from build123d import *

# Parameters (mm, degrees)
F0_R      = 6
F1_DEPTH  = 1
F2_R      = 12
F2_R_2    = 6
F3_DEPTH  = 10.5
F5_DEPTH  = 10.5
F6_R      = 4
F7_DEPTH  = 6.5
F8_R      = 3
F9_DEPTH  = 8.382
F10_W     = 2.7
F10_H     = 0.5
F11_DEPTH = 3.5
F12_R     = 16.3576
F13_DEPTH = 16.51


with BuildPart() as f1:
    # F0 (on Top) → F1 (new body)
    with BuildSketch(Plane.XY):
        Circle(F0_R)
    extrude(amount=-F1_DEPTH)

    # F2 (on face) → F3 (join)
    with BuildSketch(Plane(origin=(0, 0, -1), x_dir=(1, 0, 0), z_dir=(0, 0, -1))):
        Circle(F2_R)
        Circle(F2_R_2, mode=Mode.SUBTRACT)
        Circle(F2_R_2)
    extrude(amount=F3_DEPTH)

    # F4 (on face) → F5 (join, through all)
    with BuildSketch(Plane.XY.offset(-1)):
        with BuildLine():
            Line((6.35, 9), (6.35, -9))
            Line((6.35, -9), (7.9372539332, -9))
            ThreePointArc((7.9372539332, -9), (10.9372539332, -4.9372539332), (12, 0))
            ThreePointArc((12, 0), (10.9372539332, 4.9372539332), (7.9372539332, 9))
            Line((7.9372539332, 9), (6.35, 9))
        make_face()
        with BuildLine():
            ThreePointArc((12, 0), (10.9372539332, -4.9372539332), (7.9372539332, -9))
            Line((7.9372539332, -9), (20, -9))
            Line((20, -9), (20, 9))
            Line((20, 9), (7.9372539332, 9))
            ThreePointArc((7.9372539332, 9), (10.9372539332, 4.9372539332), (12, 0))
        make_face()
    extrude(amount=-F5_DEPTH)

    # F6 (on face) → F7 (join)
    with BuildSketch(Plane.XY):
        Circle(F6_R)
    extrude(amount=F7_DEPTH)

    # F8 (on face) → F9 (join)
    with BuildSketch(Plane.XY.offset(6.5)):
        Circle(F8_R)
    extrude(amount=F9_DEPTH)

    # F10 (on face) → F11 (join)
    with BuildSketch(Plane.XY.offset(-1)):
        with Locations((0, -12)):
            Rectangle(F10_W, F10_H)
    extrude(amount=F11_DEPTH)

    # F12 (on face) → F13 (join)
    with BuildSketch(Plane.XY.offset(6.5)):
        Circle(F12_R)
    extrude(amount=F13_DEPTH)


solid = f1.part
Check sheet for the modelled part. Datum: model origin and axes. Units: mm. A direction names the side the tool comes from. Round coordinates to 2 decimals unless told otherwise and drop trailing zeros. Loops run counter-clockwise (first coordinate to the right, second up) from the corner with the lowest first, then second, coordinate; pieces in that order, holes last. Notation, with made-up numbers: (59, -33) - (81, -33) arc R13 ccw to (81, -23) - close; hole circle Ø10 at (29.25, -7). An arc over 180 degrees is marked (long way). Answer as CSV lines item,"result". Start each with the question number.
Item 1: Section check B-B (y = -11). Record the boundary of the cut face in (x, z), and give its area (3 significant figures).
Item 2: Section check C-C (x = 0.5). Record the boundary of the cut face in (y, z).
Item 3: Section check D-D (x = 6.5). Record the boundary of the cut face in (y, z), and give its area (3 significant figures).
Item 4: Section check A-A (y = 0). Record the boundary of the cut face in (x, z).
Item 5: Release check for a two-part mould opening along Z. For faces 5 (the flat face through (-1.42, -3.92, 0)), 6 (the flat face through (0, 0, 23.01)), 7 (the flat face through (4, 0, -11.5)) record: +Z half, -Z half, draft (parallel to the pull), parting line (faces both ways), or undercut.
Item 6: Scan lines: line 1 (Z direction, x = -5, y = 1.5); line 2 (Z direction, x = 13.5, y = 6.5); line 3 (Z direction, x = 0, y = 13). Record each from-to range of solid material in increasing order. Write a range as [from, to].
Item 7: Set-up check for faces 1 (the flat face through (0, -12.25, 1)), 2 (the cylindrical face through (-12, 0, -6)), 3 (the cylindrical face through (15.602, 4.913, 14.639)), 4 (the cylindrical face through (-5.994, 0.264, -0.493)): record each of +Z, -Z, +X, -X, +Y, -Y from which the full face is reachable in a straight line by a thin tool's end or side.
Item 8: Depth check by flat-ended pin: P1, Ø2, axis at x = 0, z = 1.5, coming from the +Y side; P2, Ø3, axis at x = 13.5, z = -6, coming from the -Y side; P3, Ø8.5, axis at x = 12, z = -6.5, coming from the +Y side. Enter the tip coordinate at first touch or a pass-through.
Report:
1,outline,"(-12.11, 6.5) - (12.11, 6.5) - (12.11, 23.01) - (-12.11, 23.01) - close; (-4.8, -11.5) - (4.8, -11.5) - (4.8, -1) - (-4.8, -1) - close"
1,area,"500 mm2"
2,outline,"(-16.35, 6.5) - (-3.97, 6.5) - (-3.97, 0) - (-5.98, 0) - (-5.98, -1) - (-11.75, -1) - (-11.75, 2.5) - (-12.25, 2.5) - (-12.25, -1) - (-11.99, -1) - (-11.99, -11.5) - (11.99, -11.5) - (11.99, -1) - (5.98, -1) - (5.98, 0) - (3.97, 0) - (3.97, 6.5) - (16.35, 6.5) - (16.35, 23.01) - (-16.35, 23.01) - close"
3,outline,"(-15.01, 6.5) - (15.01, 6.5) - (15.01, 23.01) - (-15.01, 23.01) - close; (-10.09, -11.5) - (10.09, -11.5) - (10.09, -1) - (-10.09, -1) - close"
3,area,"707 mm2"
4,outline,"(-16.36, 6.5) - (-4, 6.5) - (-4, 0) - (-6, 0) - (-6, -1) - (-12, -1) - (-12, -11.5) - (20, -11.5) - (20, -1) - (6, -1) - (6, 0) - (4, 0) - (4, 6.5) - (16.36, 6.5) - (16.36, 23.01) - (-16.36, 23.01) - close"
5,face 5,"undercut"
5,face 6,"+Z half"
5,face 7,"-Z half"
6,line 1,"z = [-11.5, 0], [6.5, 23.01]"
6,line 2,"z = [-11.5, -1], [6.5, 23.01]"
6,line 3,"z = [6.5, 23.01]"
7,face 1,"-Z, +X, -X, -Y"
7,face 2,"-Z"
7,face 3,"+Z"
7,face 4,"none"
8,P1,"stops at y = 4"
8,P2,"stops at y = -9"
8,P3,"stops at y = 9.16"
